The model under review builds one solid part; all positions refer to its coordinate system, in mm. Round coordinates to 2 decimals unless told otherwise and drop trailing zeros. Order: outer loops, then holes, each group sorted by start corner. A loop starts at its lowest first (then second) coordinate and runs counter-clockwise, first axis right, second up.
1) Consider section D-D (y = -26). Give the boundary of the cut face in (x, z).
2) Clearance check with flat-ended pins moving along their axes: P1, Ø1.5, axis at x = 27.5, z = 3, coming from the -Y side; P2, Ø1, axis at x = -4, z = 1, coming from the -Y side; P3, Ø3, axis at x = 25, y = -9, coming from the +Z side; P4, Ø0.9, axis at y = -22, z = 3, coming from the -X side. State where each tip first meets the part, or that it passes through.
3) Consider section C-C (x = 20.99). Give the boundary of the cut face in (y, z).
4) To check wall thickness, follow L1, parallel to Y at x = 5, z = 2.2; L2, parallel to X at y = -9.5, z = 0.45; L3, parallel to Y at x = 25, z = 2.25. State the ranges of each line that lie inside material, in increasing order.
5) Consider section A-A (y = -9). Give the boundary of the cut face in (x, z), then the cut area to 3 significant figures.
6) Consider section B-B (z = 2.35). Give the boundary of the cut face in (x, y), then the cut area to 3 significant figures.
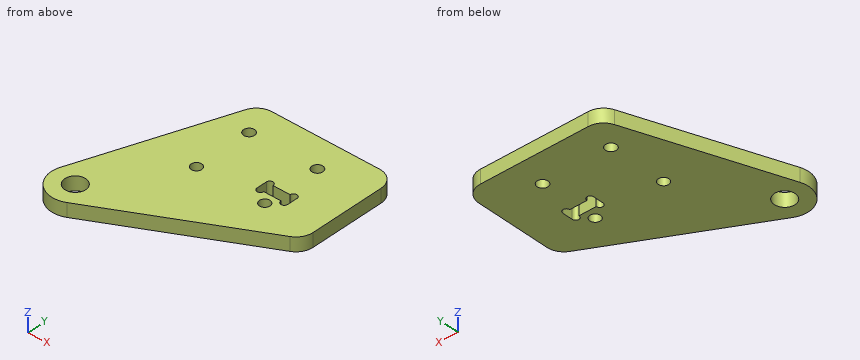
from build123d import *

# Parameters (mm, degrees)
SKETCH_1_R          = 1.6
EXTRUDE_1_DEPTH     = 4
FILLET_1_R          = 7
SKETCH_2_R          = 3.05
CUT_EXTRUDE_1_DEPTH = 5.5
FILLET_2_R          = 5
SKETCH_4_R          = 1.55
CUT_EXTRUDE_3_DEPTH = 5


with BuildPart() as part:
    # 草图1 → 凸台-拉伸1 (new body)
    with BuildSketch(Plane.XY):
        Polygon((0, 0), (40, 0), (40, -30), (-22.930124759, -63), align=None)
        with Locations((5, -9)):
            Circle(SKETCH_1_R, mode=Mode.SUBTRACT)
        with Locations((25, -9)):
            Circle(SKETCH_1_R, mode=Mode.SUBTRACT)
    extrude(amount=EXTRUDE_1_DEPTH)

    # 圆角1
    fillet_1_edges = [part.edges().sort_by_distance(p)[0] for p in [
        (-22.930124759, -63, 2),
    ]]
    fillet(fillet_1_edges, radius=FILLET_1_R)

    # 草图2 → 切除-拉伸1 (cut)
    with BuildSketch(Plane.XY.offset(4)):
        with Locations((-10.168271669, -48.403727607)):
            Circle(SKETCH_2_R)
    extrude(amount=-CUT_EXTRUDE_1_DEPTH, mode=Mode.SUBTRACT)

    # 圆角2
    fillet_2_edges = [part.edges().sort_by_distance(p)[0] for p in [
        (0, 0, 2),
        (40, 0, 2),
        (40, -30, 2),
    ]]
    fillet(fillet_2_edges, radius=FILLET_2_R)

    # 草图4 → 切除-拉伸3 (cut)
    with BuildSketch(Plane(origin=(0, 0, 0), x_dir=(-1, 0, 0), z_dir=(0, 0, -1))):
        with Locations((-25, -26)):
            Circle(SKETCH_4_R)
        with Locations((-5, -26)):
            Circle(SKETCH_4_R)
        with BuildLine():
            Line((-21.99, -23), (-27, -23))
            ThreePointArc((-27, -23), (-28, -24), (-29, -23))
            Line((-29, -23), (-29, -19.99))
            ThreePointArc((-29, -19.99), (-28, -18.99), (-27, -19.99))
            Line((-27, -19.99), (-21.99, -19.99))
            ThreePointArc((-21.99, -19.99), (-20.99, -18.99), (-19.99, -19.99))
            Line((-19.99, -19.99), (-19.99, -23))
            ThreePointArc((-19.99, -23), (-20.99, -24), (-21.99, -23))
        make_face()
    extrude(amount=-CUT_EXTRUDE_3_DEPTH, mode=Mode.SUBTRACT)


solid = part.part
Answer below:
1. outline: (-9.46, 0) - (3.45, 0) - (3.45, 4) - (-9.46, 4) - close; (6.55, 0) - (23.45, 0) - (23.45, 4) - (6.55, 4) - close; (26.55, 0) - (40, 0) - (40, 4) - (26.55, 4) - close
2. P1: stops at y = -36.95
2. P2: stops at y = -53.34
2. P3: passes through
2. P4: stops at x = -8.17
3. outline: (-39.97, 0) - (-24, 0) - (-24, 4) - (-39.97, 4) - close; (-18.99, 0) - (0, 0) - (0, 4) - (-18.99, 4) - close
4. L1: y = -48.35 to -27.55, -24.45 to -10.6, -7.4 to 0
4. L2: x = -3.46 to 3.48, 6.52 to 23.48, 26.52 to 40
4. L3: y = -37.87 to -27.55, -24.45 to -23, -19.99 to -10.6, -7.4 to 0
5. outline: (-3.28, 0) - (3.4, 0) - (3.4, 4) - (-3.28, 4) - close; (6.6, 0) - (23.4, 0) - (23.4, 4) - (6.6, 4) - close; (26.6, 0) - (40, 0) - (40, 4) - (26.6, 4) - close
5. area: 148 mm2
6. outline: (-16.75, -46.01) arc R7 ccw to (-6.92, -54.6) - (37.32, -31.4) arc R5 ccw to (40, -26.98) - (40, -5) arc R5 ccw to (35, 0) - (3.5, 0) arc R5 ccw to (-1.2, -3.29) - close; hole circle Ø6.1 at (-10.17, -48.4); hole circle Ø3.2 at (5, -9); hole circle Ø3.1 at (5, -26); hole (19.99, -23) arc R1 ccw to (21.99, -23) - (27, -23) arc R1 ccw to (29, -23) - (29, -19.99) arc R1 ccw to (27, -19.99) - (21.99, -19.99) arc R1 ccw to (19.99, -19.99) - close; hole circle Ø3.2 at (25, -9); hole circle Ø3.1 at (25, -26)
6. area: 2,030 mm2
